from build123d import *

# Parameters (mm, degrees)
BOSS_EXTRUDE1_DEPTH = 25.4
SKETCH2_R           = 7.62
BOSS_EXTRUDE2_DEPTH = 1.27
SKETCH3_R           = 1.27
CUT_EXTRUDE1_DEPTH  = 1.27


with BuildPart() as part:
    # Sketch1 → Boss-Extrude1 (new body)
    with BuildSketch(Plane.XY):
        with BuildLine():
            Line((-17.78, 12.7), (17.78, 12.7))
            ThreePointArc((17.78, 12.7), (23.168153673, 10.468153673), (25.4, 5.08))
            Line((25.4, 5.08), (25.4, -5.08))
            ThreePointArc((25.4, -5.08), (23.168153673, -10.468153673), (17.78, -12.7))
            Line((17.78, -12.7), (-17.78, -12.7))
            ThreePointArc((-17.78, -12.7), (-23.168153673, -10.468153673), (-25.4, -5.08))
            Line((-25.4, -5.08), (-25.4, 5.08))
            ThreePointArc((-25.4, 5.08), (-23.168153673, 10.468153673), (-17.78, 12.7))
        make_face()
    extrude(amount=BOSS_EXTRUDE1_DEPTH)

    # Sketch2 → Boss-Extrude2 (add)
    with BuildSketch(Plane.XY.offset(25.4)):
        with Locations(Location((12.7, 0, 0), (0, 0, 180))):
            Circle(SKETCH2_R)
    extrude(amount=BOSS_EXTRUDE2_DEPTH)

    # Sketch3 → Cut-Extrude1 (cut)
    with BuildSketch(Plane.XY.offset(26.67)):
        with Locations((12.7, 0)):
            Circle(SKETCH3_R)
    extrude(amount=-CUT_EXTRUDE1_DEPTH, mode=Mode.SUBTRACT)


solid = part.part
Input: part model. Units: mm. Frame: model coordinates. A direction names the side the tool comes from. Give positions to 0.01 mm unless a question says otherwise; leave off trailing zeros. Order: outer loops, then holes, each group sorted by start corner. A loop starts at its lowest first (then second) coordinate and runs counter-clockwise, first axis right, second up. Notation, with made-up numbers: (72, 41.25) - (91, 41.25) arc R20 ccw to (91, 45.25) - close; hole circle Ø2 at (68.25, 75.25). An arc over 180 degrees is marked (long way). Answer as a JSON object with one key per item and string values. Group by question number.
Q1. First-contact query: pin 1 Ø1.5 at (x, y) = (-7.5, -7) entering from +Z; pin 2 Ø12 at (x, y) = (6.5, -10) entering from +Z; pin 3 Ø1 at (y, z) = (7.5, 18) entering from -X. Flat tips, straight axial feed; report the tip coordinate or a pass-through.
Q2. Cut plane A-A, the plane x = 12.7. Output: boundary loops of the cut face in (y, z).
Q3. Set-up query: faces 5 (the face through (5.432, -2.289, 26.026)), 6 (the face through (-23.109, -10.527, 12.522)). Return all of +Z, -Z, +X, -X, +Y, -Y with unobstructed straight access to the full face (end or side cutting, diameter ignored); none if empty.
Q4. Cut plane B-B, the plane y = 0. Output: boundary loops of the cut face in (x, z).
Q5. Line query: probe 1 along Y at (x, z) = (12.7, 25.95); probe 2 along Z at (x, y) = (-6, 7.5); probe 3 along X at (y, z) = (-11, 12.75). Output: solid intervals per line, ascending.
Q6. Mould query, pull axis Y, two halves, no side actions, for faces 1 (the face through (0, 12.7, 13)), 2 (the face through (0, 0, 0)), 3 (the face through (13, 0, 25.4)), 4 (the face through (13.87, -0.49, 26.04)). Classes: pulls with the +Y half, pulls with the -Y half, needs draft (parallel to the pull), parting line crosses it, or undercut.
Q7. Cut plane D-D, the plane y = -4. Output: boundary loops of the cut face in (x, z), then the cut area to 3 significant figures.
Q8. Cut plane C-C, the plane z = 5.5. Output: boundary loops of the cut face in (x, y).
Results:
{
 "1": {"pin 1": "z = 25.4", "pin 2": "z = 26.67", "pin 3": "x = -25.15"},
 "2": {"outline": "(-12.7, 0) - (12.7, 0) - (12.7, 25.4) - (7.62, 25.4) - (7.62, 26.67) - (1.27, 26.67) - (1.27, 25.4) - (-1.27, 25.4) - (-1.27, 26.67) - (-7.62, 26.67) - (-7.62, 25.4) - (-12.7, 25.4) - close"},
 "3": {"face 5": "+Z", "face 6": "+Z, -Z, -X, -Y"},
 "4": {"outline": "(-25.4, 0) - (25.4, 0) - (25.4, 25.4) - (20.32, 25.4) - (20.32, 26.67) - (13.97, 26.67) - (13.97, 25.4) - (11.43, 25.4) - (11.43, 26.67) - (5.08, 26.67) - (5.08, 25.4) - (-25.4, 25.4) - close"},
 "5": {"probe 1": "-7.62 to -1.27, 1.27 to 7.62", "probe 2": "0 to 25.4", "probe 3": "-22.58 to 22.58"},
 "6": {"face 1": "pulls with the +Y half", "face 2": "needs draft", "face 3": "undercut", "face 4": "undercut"},
 "7": {"outline": "(-25.4, 0) - (25.4, 0) - (25.4, 25.4) - (19.19, 25.4) - (19.19, 26.67) - (6.21, 26.67) - (6.21, 25.4) - (-25.4, 25.4) - close", "area": "1,310 mm^2"},
 "8": {"outline": "(-25.4, -5.08) arc R7.62 ccw to (-17.78, -12.7) - (17.78, -12.7) arc R7.62 ccw to (25.4, -5.08) - (25.4, 5.08) arc R7.62 ccw to (17.78, 12.7) - (-17.78, 12.7) arc R7.62 ccw to (-25.4, 5.08) - close"}
}
